```python
from build123d import *

# Parameters (mm, degrees)
SKETCH1_W           = 30
SKETCH1_H           = 10
BOSS_EXTRUDE1_DEPTH = 10.5
SKETCH3_W           = 2
SKETCH3_H           = 6
CUT_EXTRUDE1_DEPTH  = 34.320414163
LPATTERN1_COUNT     = 13
LPATTERN1_PITCH     = 2


with BuildPart() as part:
    # Sketch1 → Boss-Extrude1 (new body)
    with BuildSketch(Plane.XY):
        with Locations((15, 5)):
            Rectangle(SKETCH1_W, SKETCH1_H)
    extrude(amount=BOSS_EXTRUDE1_DEPTH)

    # Sketch3 → Cut-Extrude1 (cut, symmetric)
    with BuildSketch(Plane.XZ):
        with Locations((3, 3)):
            Rectangle(SKETCH3_W, SKETCH3_H)
    cut_extrude1 = extrude(amount=CUT_EXTRUDE1_DEPTH, both=True, mode=Mode.SUBTRACT)

    # LPattern1: Cut-Extrude1 ×13, 6 skipped
    with Locations(*[(i * LPATTERN1_PITCH, 0, 0) for i in range(1, LPATTERN1_COUNT) if i not in (1, 3, 5, 7, 9, 11)]):
        add(cut_extrude1, mode=Mode.SUBTRACT)


solid = part.part
```
For this review, take the finished solid that the model builds, in its own axes (mm). A direction names the side the tool comes from. Round coordinates to 2 decimals unless told otherwise and drop trailing zeros. Write each loop counter-clockwise with the first axis right and the second up, starting at its lowest first coordinate (ties: lowest second). Pieces come first, ordered by that corner, then holes. Notation, with made-up numbers: (-16, 15) - (-6, 15) arc R29 cw to (-6, 44) - close; hole circle Ø1 at (76, 50). An arc over 180 degrees is marked (long way). Answer as CSV lines item,"result". Start each with the question number.
(1) Mouldability with a two-part tool opening along X and no side actions: class faces 1 (the flat face through (15, 5, 6)), 2 (the flat face through (13, 5, 0)), 3 (the flat face through (16, 5, 3)), 4 (the flat face through (0, 5, 5)) as +X half, -X half, draft (parallel to the pull), parting line (faces both ways), or undercut.
(2) Machinability: for faces 5 (the flat face through (14.8, 0, 6.3)), 6 (the flat face through (4, 5, 3)), which of the approach directions +Z, -Z, +X, -X, +Y, -Y give a long, thin tool a straight path to every point of the face, cutting with its end or side? Answer none if there is none.
(3) Add section C-C, the plane x = 26.5. State the section outline as (y, z) points, plus the area to 3 significant figures.
(4) For line 1 (Z direction, x = 2.75, y = 2.5), list the stretches that pass through material, from the lowest coordinate up.
(5) Add section A-A, the plane z = 1.25. State how many separate pieces and enclosed holes the cut face has, plus the area to 3 significant figures.
From the geometry:
1,face 1,"undercut"
1,face 2,"draft"
1,face 3,"undercut"
1,face 4,"-X half"
2,face 5,"+Z, -Z, +X, -X, -Y"
2,face 6,"-Z, +Y, -Y"
3,outline,"(0, 6) - (10, 6) - (10, 10.5) - (0, 10.5) - close"
3,area,"45.0 mm²"
4,line 1,"z = 6 to 10.5"
5,separate pieces,"8"
5,enclosed holes,"0"
5,area,"160 mm²"
